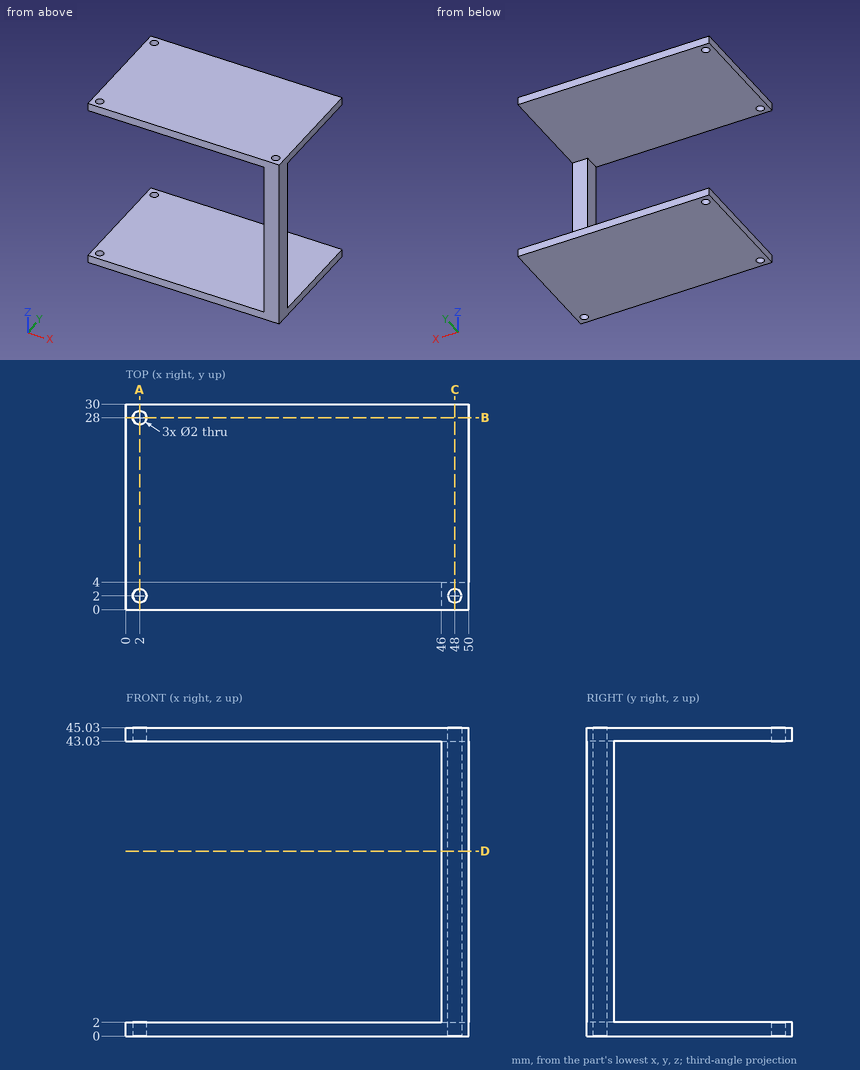
Geometry check sheet. Reference: drawing and pictorial views, mm from the part's lowest x, y, z. Give positions to 0.01 mm unless a question says otherwise; leave off trailing zeros. Order: outer loops, then holes, each group sorted by start corner. A loop starts at its lowest first (then second) coordinate and runs counter-clockwise, first axis right, second up. Notation, with made-up numbers: M 27.5,8.25 L 63.5,8.25 A28 ccw 63.5,37.25 Z; hole C 26,-37 d9. An arc over 180 degrees is marked long. Answer in a Markdown table with one row per item. Add a question column.
Item 1: Scan lines: probe 1 along Y at (x, z) = (2, 0.55); probe 2 along Z at (x, y) = (5, 18); probe 3 along Y at (x, z) = (48, 18). Record each from-to range of solid material in increasing order. Write a range as from..to.
Item 2: Section check B-B, the plane y = 28. Enter the section's corners in (x, z).
Item 3: Section check D-D, the plane z = 27. Enter the section's corners in (x, y).
Item 4: Section check A-A, the plane x = 2. Enter the section's corners in (y, z).
Item 5: Section check C-C, the plane x = 48. Enter the section's corners in (y, z).
Item 6: Gauge pin test, flat ends, axial feed: pin 1 (3 mm diameter, centred on x = 47.5, z = 13.5, fed in from +Y); pin 2 (4.5 mm diameter, centred on y = 2.5, z = 21.5, fed in from -X). Record the tip position at first contact, or that the pin passes through.
Filled sheet:
| question | item | result |
|---|---|---|
| 1 | probe 1 | y = 0..1, 3..27, 29..30 |
| 1 | probe 2 | z = 0..2, 43.03..45.03 |
| 1 | probe 3 | y = 0..1, 3..4 |
| 2 | outline | M 0,0 L 1,0 L 1,2 L 0,2 Z; M 0,43.03 L 1,43.03 L 1,45.03 L 0,45.03 Z; M 3,0 L 50,0 L 50,2 L 3,2 Z; M 3,43.03 L 50,43.03 L 50,45.03 L 3,45.03 Z |
| 3 | outline | M 46,0 L 50,0 L 50,4 L 46,4 Z; hole C 48,2 d2 |
| 4 | outline | M 0,0 L 1,0 L 1,2 L 0,2 Z; M 0,43.03 L 1,43.03 L 1,45.03 L 0,45.03 Z; M 3,0 L 27,0 L 27,2 L 3,2 Z; M 3,43.03 L 27,43.03 L 27,45.03 L 3,45.03 Z; M 29,0 L 30,0 L 30,2 L 29,2 Z; M 29,43.03 L 30,43.03 L 30,45.03 L 29,45.03 Z |
| 5 | outline | M 0,0 L 1,0 L 1,45.03 L 0,45.03 Z; M 3,0 L 30,0 L 30,2 L 4,2 L 4,43.03 L 30,43.03 L 30,45.03 L 3,45.03 Z |
| 6 | pin 1 | stops at y = 4 |
| 6 | pin 2 | stops at x = 46 |
